from build123d import *

# Parameters (mm, degrees)
BOSS_EXTRUDE1_DEPTH = 0.254
SKETCH2_R           = 4.699
CUT_EXTRUDE1_DEPTH  = 1.254
SKETCH3_W           = 2.54
SKETCH3_H           = 0.635
CUT_EXTRUDE2_DEPTH  = 1.254
SKETCH5_OUTSIDE_W   = 121.447
SKETCH5_OUTSIDE_H   = 109.618
CUT_EXTRUDE5_DEPTH  = 1.254


with BuildPart() as part:
    # Sketch1 → Boss-Extrude1 (new body)
    with BuildSketch(Plane.XY):
        with BuildLine():
            Line((67.21146711, 76.191723231), (8.696654013, 17.676910134))
            Line((8.696654013, 17.676910134), (7.228954972, 14.133571205))
            ThreePointArc((7.228954972, 14.133571205), (14.666587579, 6.075099489), (15.105587123, -4.88230096))
            Line((15.105587123, -4.88230096), (18.648926052, -6.35))
            Line((18.648926052, -6.35), (101.401368334, -6.35))
            ThreePointArc((101.401368334, -6.35), (93.866160503, 38.880636728), (67.21146711, 76.191723231))
        make_face()
        with BuildLine():
            Line((88.672924278, 6.35), (27.86051193, 6.35))
            ThreePointArc((27.86051193, 6.35), (26.399857642, 10.93517908), (24.190484974, 15.210228852))
            Line((24.190484974, 15.210228852), (67.191354125, 58.211098004))
            ThreePointArc((67.191354125, 58.211098004), (82.13289044, 34.020557137), (88.672924278, 6.35))
        make_face(mode=Mode.SUBTRACT)
    extrude(amount=BOSS_EXTRUDE1_DEPTH)

    # Sketch2 → Cut-Extrude1 (cut, through all)
    with BuildSketch(Plane.XY.offset(0.254)):
        with Locations((22.225, 0)):
            Circle(SKETCH2_R)
        with Locations((36.195, 0)):
            Circle(SKETCH2_R)
        with Locations((61.722, 0)):
            Circle(SKETCH2_R)
        with Locations((75.692, 0)):
            Circle(SKETCH2_R)
        with Locations((95.25, 0)):
            Circle(SKETCH2_R)
        with Locations((15.715448212, 15.715448212)):
            Circle(SKETCH2_R)
        with Locations((25.593729945, 25.593729945)):
            Circle(SKETCH2_R)
        with Locations((43.644044748, 43.644044748)):
            Circle(SKETCH2_R)
        with Locations((53.522326482, 53.522326482)):
            Circle(SKETCH2_R)
        with Locations((92.004434954, 24.652514046)):
            Circle(SKETCH2_R)
        with Locations((82.48891971, 47.625)):
            Circle(SKETCH2_R)
        with Locations((67.351920908, 67.351920908)):
            Circle(SKETCH2_R)
    extrude(amount=-CUT_EXTRUDE1_DEPTH, mode=Mode.SUBTRACT)

    # Sketch3 → Cut-Extrude2 (cut, through all)
    with BuildSketch(Plane.XY.offset(0.254)):
        Polygon((15.266435406, 24.246691527), (17.06248663, 26.042742751), (17.511499436, 25.593729945), (15.715448212, 23.797678721), align=None)
        Polygon((44.991083167, 53.971339288), (43.195031942, 52.175288063), (43.644044748, 51.726275257), (45.440095973, 53.522326482), align=None)
        with Locations((29.21, -6.0325)):
            Rectangle(SKETCH3_W, SKETCH3_H)
        with Locations((68.707, -6.0325)):
            Rectangle(SKETCH3_W, SKETCH3_H)
        Polygon((29.230733674, 38.210989795), (31.026784898, 40.007041019), (31.475797704, 39.558028213), (29.67974648, 37.761976989), align=None)
        Polygon((56.845021246, 65.825277367), (55.048970022, 64.029226143), (55.497982828, 63.580213337), (57.294034052, 65.376264561), align=None)
        with Locations((48.9585, -6.0325)):
            Rectangle(SKETCH3_W, SKETCH3_H)
        with Locations((85.471, -6.0325)):
            Rectangle(SKETCH3_W, SKETCH3_H)
        Polygon((99.935462164, 14.437711971), (100.266998693, 11.919442024), (101.526133667, 12.085210288), (101.194597138, 14.603480236), align=None)
        Polygon((93.765504959, 37.464305742), (94.938831965, 37.950313702), (93.966816047, 40.296967714), (92.793489041, 39.810959755), align=None)
        Polygon((79.327792988, 62.471156422), (80.874047017, 60.456038938), (81.88160576, 61.229165953), (80.33535173, 63.244283437), align=None)
        Polygon((13.593916116, 7.005422516), (14.565932035, 4.658768503), (15.739259041, 5.144776462), (14.767243123, 7.491430475), align=None)
    extrude(amount=-CUT_EXTRUDE2_DEPTH, mode=Mode.SUBTRACT)

    # Sketch5 outside → Cut-Extrude5 (cut, through all)
    with BuildSketch(Plane.XY.offset(0.254)):
        with Locations((54.4145, 34.921)):
            Rectangle(SKETCH5_OUTSIDE_W, SKETCH5_OUTSIDE_H)
        with BuildLine():
            Line((70.287378691, 52.332602618), (82.379165395, 61.610956889))
            ThreePointArc((82.379165395, 61.610956889), (89.088033287, 51.435), (94.546236515, 40.53697153))
            Line((94.546236515, 40.53697153), (80.465052659, 34.704354203))
            ThreePointArc((80.465052659, 34.704354203), (75.889806134, 43.815), (70.287378691, 52.332602618))
        make_face(mode=Mode.SUBTRACT)
    extrude(amount=-CUT_EXTRUDE5_DEPTH, mode=Mode.SUBTRACT)


solid = part.part
The listing builds one solid part. Answer for the finished solid, in the listing's coordinates (mm). Round coordinates to 2 decimals unless told otherwise and drop trailing zeros. Order: outer loops, then holes, each group sorted by start corner. A loop starts at its lowest first (then second) coordinate and runs counter-clockwise, first axis right, second up. Notation, with made-up numbers: (60.25, 69) -> (106.25, 69) arc R5 cw to (106.25, 78) -> close; hole circle Ø8 at (-39.5, 23.25). An arc over 180 degrees is marked (long way). Put each result on its own line as item: value.
Q1. Section B-B, the plane y = 46 is taken. Write down the section's boundary in (x, z).
Results list:
outline: (76.07, 0) -> (78.08, 0) -> (78.08, 0.25) -> (76.07, 0.25) -> close; (86.9, 0) -> (90.59, 0) -> (90.59, 0.25) -> (86.9, 0.25) -> close
Q2. Section A-A, the plane x = 79 is taken. Write down the section's boundary in (y, z).
Results list:
outline: (40.77, 0) -> (44.48, 0) -> (44.48, 0.25) -> (40.77, 0.25) -> close; (50.77, 0) -> (59.02, 0) -> (59.02, 0.25) -> (50.77, 0.25) -> close
Q3. Section C-C, the plane z = 0.2 is taken. Write down the section's boundary in (x, y) (1 decimal).
Results list:
outline: (71.3, 53.1) arc R88.9 cw to (81.6, 35.2) -> (93.4, 40.1) arc R101.6 ccw to (81.4, 60.8) -> close; hole circle Ø9.4 at (82.5, 47.6)
Q4. This flat-tipped pin is pushed along its axis until it touches: P1, Ø7.5, axis at x = 82.49, y = 47.62, coming from the -Z side. Where does it stop, or does it pass through?
Results list:
P1: through
Q5. Consider line 1 along Y through (x, z) = (86.25, 0.2); line 2 along Y through (x, z) = (81.5, 0.15); line 3 along X through (y, z) = (50.75, 0.2). Determine where each line is inside the solid, lowest interval first.
Results list:
line 1: 37.1 to 44.81, 50.44 to 53.7
line 2: 35.51 to 43.03, 52.22 to 60.67
line 3: 72.99 to 78.98, 86 to 88.02
Q6. Section D-D, the plane y = 58.75 is taken. Write down the section's boundary in (x, z), and give its area (3 significant figures).
Results list:
outline: (78.65, 0) -> (82.89, 0) -> (82.89, 0.25) -> (78.65, 0.25) -> close
area: 1.08 mm^2
